from build123d import *

# Parameters (mm, degrees)
F0_R     = 50
F0_R_2   = 46
F0_R_3   = 42
F1_DEPTH = 5
F2_DEPTH = 500
F3_DEPTH = 35
F4_R     = 7


with BuildPart() as f1:
    # F0 (on Top) → F1 (new body)
    with BuildSketch(Plane.XY):
        Circle(F0_R)
        Circle(F0_R_2, mode=Mode.SUBTRACT)
        Circle(F0_R_2)
        Circle(F0_R_3, mode=Mode.SUBTRACT)
        Circle(F0_R_3)
    extrude(amount=F1_DEPTH)

    # F0 (on Top) → F2 (join)
    with BuildSketch(Plane.XY):
        Circle(F0_R_2)
        Circle(F0_R_3, mode=Mode.SUBTRACT)
    extrude(amount=-F2_DEPTH)

    # F0 (on Top) → F3 (join)
    with BuildSketch(Plane.XY):
        Circle(F0_R)
        Circle(F0_R_2, mode=Mode.SUBTRACT)
    extrude(amount=-F3_DEPTH)

    # F4
    f4_edges = [f1.edges().sort_by_distance(p)[0] for p in [
        (-50, 0, 5),
    ]]
    fillet(f4_edges, radius=F4_R)


solid = f1.part
Verification items for the finished model (mm, model axes). A direction names the side the tool comes from. Coordinates: 2 decimals unless noted, no trailing zeros. Order: outer loops, then holes, each group sorted by start corner. A loop starts at its lowest first (then second) coordinate and runs counter-clockwise, first axis right, second up. Notation, with made-up numbers: M 62,-19.5 L 120,-19.5 A20 cw 120,-12.5 Z; hole C -7,28 d8. An arc over 180 degrees is marked long. One line per item, written item: value. Start each with the question number.
Item 1: Depth check by flat-ended pin: P1, Ø25, axis at x = 3.5, y = 5, coming from the -Z side; P2, Ø1, axis at y = -7, z = -152, coming from the -X side; P3, Ø1, axis at y = 30.5, z = -253.5, coming from the +X side. Enter the tip coordinate at first touch or a pass-through.
Item 2: Thickness scan on probe 1 along Y at (x, z) = (0, -114); probe 2 along Z at (x, y) = (10, -22); probe 3 along Y at (x, z) = (14.5, -146). Record the ranges inside material, lowest first.
Item 3: Sectioned sample at B-B on z = -356.5. Record the cut outline in (x, y).
Item 4: Sectioned sample at A-A on x = 0. Record the cut outline in (y, z).
Item 5: Access from +Z, -Z, +X, -X, +Y, -Y to the whole of each face (thin tool, end or side, straight path). Record for faces 1 (the flat face through (20.2, -37.3, -500)), 2 (the cylindrical face through (-5.99, 45.61, -264.24)).
Item 6: Mould release check, pull along Y, two halves, no side actions. Record for faces 3 (the cylindrical face through (40.06, 12.62, -246.5)), 4 (the cylindrical face through (47.69, 15.02, -18.27)), 5 (the flat face through (-1, 1, 5)), 6 (the flat face through (-1, 1, 0)): pulls with the +Y half, pulls with the -Y half, needs draft (parallel to the pull), parting line crosses it, or undercut.
Calculated:
1. P1: z = 0
1. P2: x = -45.54
1. P3: x = 34.87
2. probe 1: -46 to -42, 42 to 46
2. probe 2: 0 to 5
2. probe 3: -43.65 to -39.42, 39.42 to 43.65
3. outline: C 0,0 d92; hole C 0,0 d84
4. outline: M -50,-35 L -46,-35 L -46,-500 L -42,-500 L -42,0 L 42,0 L 42,-500 L 46,-500 L 46,-35 L 50,-35 L 50,-2 A7 ccw 43,5 L -43,5 A7 ccw -50,-2 Z
5. face 1: -Z, +X, -X, +Y, -Y
5. face 2: -Z
6. face 3: undercut
6. face 4: parting line crosses it
6. face 5: needs draft
6. face 6: undercut
